Part print with two shaded views. Sizes in mm from the minimum x, y, z corner. Coordinates: 2 decimals unless noted, no trailing zeros. Loops run counter-clockwise (first coordinate to the right, second up) from the corner with the lowest first, then second, coordinate; pieces in that order, holes last. Notation, with made-up numbers: (33.25, 56) - (50.25, 56) arc R17 cw to (50.25, 71) - close; hole circle Ø7 at (67, 36). An arc over 180 degrees is marked (long way). Answer as CSV lines item,"result".
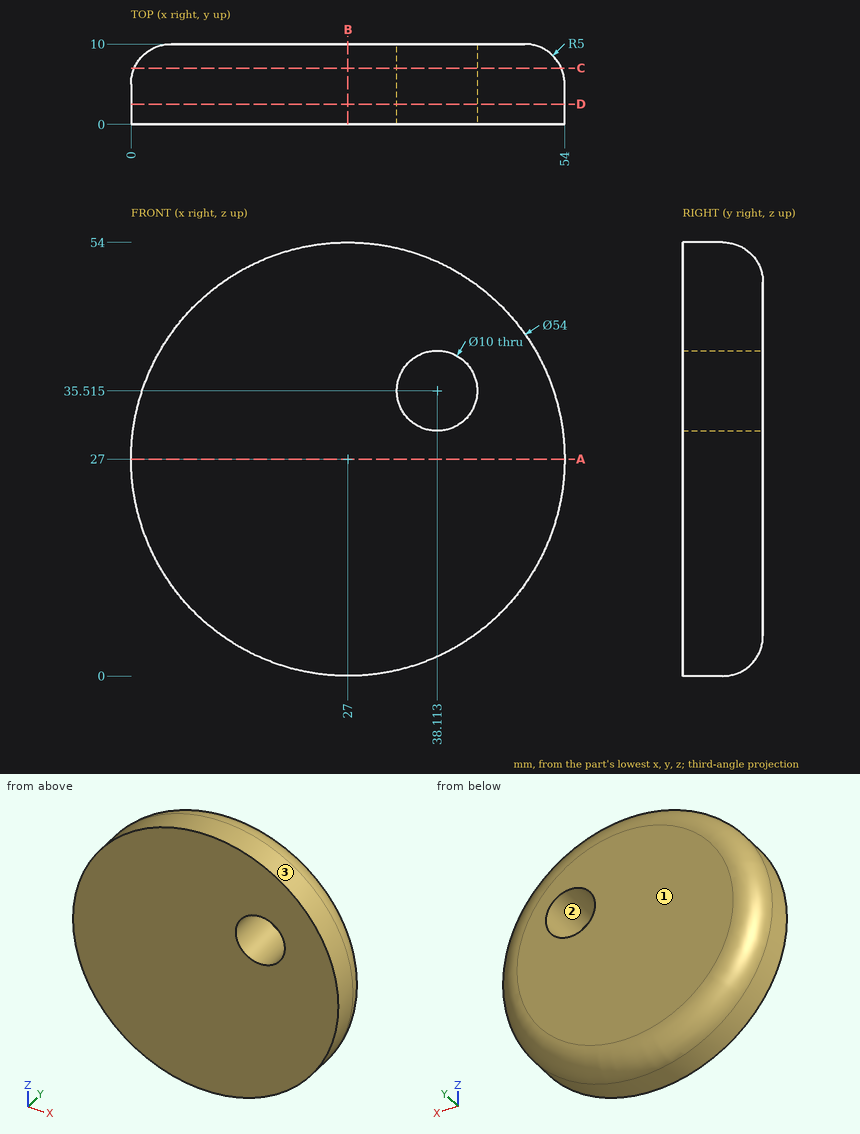
Q1. Saw through at B-B (x = 27). Give the cut face in (y, z).
Results:
outline,"(0, 0) - (5, 0) arc R5 ccw to (10, 5) - (10, 49) arc R5 ccw to (5, 54) - (0, 54) - close"
Q2. Flat gauge pins, fed straight in: pin 1 (3 mm diameter, centred on x = 32, y = 8, fed in from +Z); pin 2 (6 mm diameter, centred on y = 8, z = 35.5, fed in from +X); pin 3 (5 mm diameter, centred on y = 3.5, z = 15.5, fed in from +X). Where does each tip first touch, or does it go through?
Results:
pin 1,"stops at z = 53.36"
pin 2,"stops at x = 53.16"
pin 3,"stops at x = 52.46"
Q3. Wall check: L1, parallel to Z at x = 34.5, y = 9.5 (1 decimal); L2, parallel to Z at x = 37, y = 6.5; L3, parallel to X at y = 5, z = 32 (1 decimal). Give the ranges that are in metal, low to high.
Results:
L1,"z = 4 to 32.1, 39 to 50"
L2,"z = 2.17 to 30.64, 40.39 to 51.83"
L3,"x = 0.5 to 34.6, 41.7 to 53.5"
Q4. Two-plate mould, pull along X, no slides. Class the marked faces 1, 2 and 3: released by +X, released by -X, zero draft, split by the parting line, or undercut.
Results:
face 1,"zero draft"
face 2,"undercut"
face 3,"split by the parting line"
Q5. Saw through at A-A (z = 27). Give the cut face in (x, y).
Results:
outline,"(0, 0) - (54, 0) - (54, 5) arc R5 ccw to (49, 10) - (5, 10) arc R5 ccw to (0, 5) - close"
Q6. Saw through at D-D (y = 2.5). Give the cut face in (x, z) (1 decimal).
Results:
outline,"circle Ø54 at (27, 27); hole circle Ø10 at (38.1, 35.5)"
Q7. Saw through at C-C (y = 7). Give the cut face in (x, z) (1 decimal).
Results:
outline,"circle Ø53.2 at (27, 27); hole circle Ø10 at (38.1, 35.5)"
